```python
from build123d import *

# Parameters (mm, degrees)
BLANKSKE_W        = 100
BLANKSKE_H        = 21.5
BLANK_DEPTH       = 10
TOOTHCUTSIM_DEPTH = 103.772807688
TEETHCUTS_COUNT   = 22
TEETHCUTS_PITCH   = 4.712388975


with BuildPart() as part:
    # BlankSke → Blank (new body)
    with BuildSketch(Plane.XY):
        with Locations((50, 10.75)):
            Rectangle(BLANKSKE_W, BLANKSKE_H)
    extrude(amount=-BLANK_DEPTH)

    # TooCutSkeSim → ToothCutSim (cut, through all)
    with BuildSketch(Plane.XY):
        Polygon((0.654653055, 18.125), (-0.654653055, 18.125), (-1.892297439, 21.5254), (1.892297439, 21.5254), align=None)
    toothcutsim = extrude(amount=-TOOTHCUTSIM_DEPTH, mode=Mode.SUBTRACT)

    # TeethCuts: ToothCutSim ×22
    with Locations(*[(i * TEETHCUTS_PITCH, 0, 0) for i in range(1, TEETHCUTS_COUNT)]):
        add(toothcutsim, mode=Mode.SUBTRACT)


solid = part.part
```
Check sheet for the modelled part. Datum: model origin and axes. Units: mm. Round coordinates to 2 decimals unless told otherwise and drop trailing zeros.
1) Section check A-A (y = 20.25). Give the number of separate pieces and of enclosed holes in the cut face, and give its area (3 significant figures).
2) Scan line: line 1 (Y direction, x = 89, z = -8.25) (3 decimals). Record every from-to range of solid material in increasing order.
3) Go/stop test with a flat-tipped pin: pin 1 Ø1 at (x, z) = (66, -5) entering from +Y (3 decimals). Record where the tip stops, or that it passes through.
4) Mould release check, pull along X, two halves, no side actions. Record for faces 1 (the flat face through (0, 9, -5)), 2 (the flat face through (49, 11, 0)), 3 (the flat face through (31.726, 19.789, -4.93)): +X half, -X half, draft (parallel to the pull), parting line (faces both ways), or undercut.
Result:
1. separate pieces: 21
1. enclosed holes: 0
1. area: 390 mm2
2. line 1: y = 0 to 18.125
3. pin 1: stops at y = 18.125
4. face 1: -X half
4. face 2: draft
4. face 3: undercut
